Can you work these out from the model? Positions are in its coordinate system, mm. Give positions to 0.01 mm unless a question says otherwise; leave off trailing zeros. Order: outer loops, then holes, each group sorted by start corner. A loop starts at its lowest first (then second) coordinate and runs counter-clockwise, first axis right, second up.
Item 1: I want a section at D-D, the plane y = -120. Count the separate pieces of the cut face and the enclosed holes in it, then the cut area to 3 significant figures.
Item 2: If we mould it in two halves opening along X, with no side actions, what happens to faces 1 (the flat face through (-1, -115, 0)), 2 (the cylindrical face through (-66.007, -117.262, 0.986))? For each: +X half, -X half, draft (parallel to the pull), parting line (faces both ways), or undercut.
Item 3: I want a section at C-C, the plane y = -90. Write out the boundary of the cut face in (x, z).
Item 4: I want a section at A-A, the plane y = -14.5. Write out the boundary of the cut face in (x, z).
Item 5: I want a section at B-B, the plane x = 77. Write out the boundary of the cut face in (y, z).
Item 6: If I drill on line 1 along Y through (x, z) = (0, 1.05); line 2 along X through (y, z) = (10.5, 0.35); line 3 along Y through (x, z) = (-49.5, 1.9), over which ranges is the centre line in solid material (lowest first)?
Autodesk Inventor part; units mm, degrees
ref_plane "YZ Plane" through (0, 0, 0) normal (1, 0, 0) x (0, 1, 0)
ref_plane "XZ Plane" through (0, 0, 0) normal (0, 1, 0) x (-1, 0, 0)
ref_plane "XY Plane" through (0, 0, 0) normal (0, 0, 1) x (1, 0, 0)
ref_plane "РабПлоскость1" through (0, 0, 0) normal (0, 0, 1) x (1, 0, 0)
sketch "Эскиз1" plane through (0, 0, 0) normal (0, 0, 1) x (1, 0, 0)
  circle A0 centre (124.164, -120) radius 4
  circle A1 centre (93.064, -120) radius 4
  circle A2 centre (61.964, -120) radius 4
  circle A3 centre (30.864, -120) radius 4
  circle A4 centre (-0.236, -120) radius 4
  circle A5 centre (-31.336, -120) radius 4
  circle A6 centre (-62.436, -120) radius 4
  circle A7 centre (-93.536, -120) radius 4
  circle A8 centre (-124.636, -120) radius 4
  circle A9 centre (124.164, -90) radius 4
  circle A10 centre (-124.636, -90) radius 4
  circle A11 centre (124.164, -60) radius 4
  circle A12 centre (-124.636, -60) radius 4
  circle A13 centre (124.164, -30) radius 4
  circle A14 centre (-124.636, -30) radius 4
  circle A15 centre (124.164, 0) radius 4
  circle A16 centre (-124.636, 0) radius 4
  circle A17 centre (124.164, 30) radius 4
  circle A18 centre (-124.636, 30) radius 4
  circle A19 centre (124.164, 60) radius 4
  circle A20 centre (-124.636, 60) radius 4
  circle A21 centre (124.164, 90) radius 4
  circle A22 centre (-124.636, 90) radius 4
  circle A23 centre (124.164, 120) radius 4
  circle A24 centre (93.064, 120) radius 4
  circle A25 centre (61.964, 120) radius 4
  circle A26 centre (30.864, 120) radius 4
  circle A27 centre (-0.236, 120) radius 4
  circle A28 centre (-31.336, 120) radius 4
  circle A29 centre (-62.436, 120) radius 4
  circle A30 centre (-93.536, 120) radius 4
  circle A31 centre (-124.636, 120) radius 4
  line L0 (115.364, 110) -> (115.364, -110)
  line L1 (115.364, -110) -> (-114.636, -110)
  line L2 (-114.636, -110) -> (-114.636, 110)
  line L3 (-114.636, 110) -> (115.364, 110)
  arc A32 (-132.636, 130) -> (-134.636, 128) centre (-132.636, 128) ccw
  line L4 (-134.636, 128) -> (-134.636, -128)
  arc A33 (-134.636, -128) -> (-132.636, -130) centre (-132.636, -128) ccw
  line L5 (-132.636, -130) -> (132.636, -130)
  arc A34 (132.636, -130) -> (134.636, -128) centre (132.636, -128) ccw
  line L6 (134.636, -128) -> (134.636, 128)
  arc A35 (134.636, 128) -> (132.636, 130) centre (132.636, 128) ccw
  line L7 (132.636, 130) -> (-132.636, 130)
  circle A36 centre (-124.636, 120) radius 4.5
  circle A37 centre (-93.536, 120) radius 4.5
  circle A38 centre (-62.436, 120) radius 4.5
  circle A39 centre (-31.336, 120) radius 4.5
  circle A40 centre (-0.236, 120) radius 4.5
  circle A41 centre (30.864, 120) radius 4.5
  circle A42 centre (61.964, 120) radius 4.5
  circle A43 centre (93.064, 120) radius 4.5
  circle A44 centre (124.164, 120) radius 4.5
  circle A45 centre (124.164, 90) radius 4.5
  circle A46 centre (124.164, 60) radius 4.5
  circle A47 centre (124.164, 30) radius 4.5
  circle A48 centre (124.164, 0) radius 4.5
  circle A49 centre (124.164, -30) radius 4.5
  circle A50 centre (124.164, -60) radius 4.5
  circle A51 centre (124.164, -90) radius 4.5
  circle A52 centre (124.164, -120) radius 4.5
  circle A53 centre (93.064, -120) radius 4.5
  circle A54 centre (61.964, -120) radius 4.5
  circle A55 centre (30.864, -120) radius 4.5
  circle A56 centre (-0.236, -120) radius 4.5
  circle A57 centre (-31.336, -120) radius 4.5
  circle A58 centre (-62.436, -120) radius 4.5
  circle A59 centre (-93.536, -120) radius 4.5
  circle A60 centre (-124.636, -120) radius 4.5
  circle A61 centre (-124.636, -90) radius 4.5
  circle A62 centre (-124.636, -60) radius 4.5
  circle A63 centre (-124.636, -30) radius 4.5
  circle A64 centre (-124.636, 0) radius 4.5
  circle A65 centre (-124.636, 30) radius 4.5
  circle A66 centre (-124.636, 60) radius 4.5
  circle A67 centre (-124.636, 90) radius 4.5
  point P0 (0, 0)
  dimension "d0" = 9
  dimension "d1" = 9
  dimension "d2" = 9
  dimension "d3" = 9
  dimension "d4" = 9
  dimension "d5" = 9
  dimension "d6" = 9
  dimension "d7" = 9
  dimension "d8" = 9
  dimension "d9" = 9
  dimension "d10" = 9
  dimension "d11" = 9
  dimension "d12" = 9
  dimension "d13" = 9
  dimension "d14" = 9
  dimension "d15" = 9
  dimension "d16" = 9
  dimension "d17" = 9
  dimension "d18" = 9
  dimension "d19" = 9
  dimension "d20" = 9
  dimension "d21" = 9
  dimension "d22" = 9
  dimension "d23" = 9
  dimension "d24" = 9
  dimension "d25" = 9
  dimension "d26" = 9
  dimension "d27" = 9
  dimension "d28" = 9
  dimension "d29" = 9
  dimension "d30" = 9
  dimension "d31" = 9
extrude "Выдавливание1" add sketch "Эскиз1" along normal blind 2 contours L7 A35 L6 A34 L5 A33 L4 A32
properties material "Алюминий 6061"
Results list:
1. separate pieces: 10
1. enclosed holes: 0
1. area: 377 mm2
2. face 1: draft
2. face 2: undercut
3. outline: (-134.64, 0) - (-129.14, 0) - (-129.14, 2) - (-134.64, 2) - close; (-120.14, 0) - (-114.64, 0) - (-114.64, 2) - (-120.14, 2) - close; (115.36, 0) - (119.66, 0) - (119.66, 2) - (115.36, 2) - close; (128.66, 0) - (134.64, 0) - (134.64, 2) - (128.66, 2) - close
4. outline: (-134.64, 0) - (-114.64, 0) - (-114.64, 2) - (-134.64, 2) - close; (115.36, 0) - (134.64, 0) - (134.64, 2) - (115.36, 2) - close
5. outline: (-130, 0) - (-110, 0) - (-110, 2) - (-130, 2) - close; (110, 0) - (130, 0) - (130, 2) - (110, 2) - close
6. line 1: y = -130 to -124.49, -115.51 to -110, 110 to 115.51, 124.49 to 130
6. line 2: x = -134.64 to -114.64, 115.36 to 134.64
6. line 3: y = -130 to -110, 110 to 130
